from build123d import *

# Parameters (mm, degrees)
BOSS_EXTRUDE1_DEPTH   = 18
F_6_0MM_DOWEL_HOLE2_D = 9
SKETCH24_R            = 8.5
CUT_EXTRUDE7_DEPTH    = 19
CUT_EXTRUDE8_DEPTH    = 23
F_6_0MM_DOWEL_HOLE3_D = 9


with BuildPart() as part:
    # Sketch1 → Boss-Extrude1 (new body, symmetric)
    with BuildSketch(Plane.XY):
        with BuildLine():
            Line((-18.027756377, 6), (-22, 6))
            Line((-22, 6), (-22, 19))
            Line((-22, 19), (-50, 19))
            Line((-50, 19), (-50, 28))
            Line((-50, 28), (-25.690465157, 28))
            ThreePointArc((-25.690465157, 28), (-13.784048752, 35.411862419), (0, 38))
            Line((0, 38), (0, 19))
            ThreePointArc((0, 19), (-11.113055385, 15.411035007), (-18.027756377, 6))
        make_face()
    boss_extrude1 = extrude(amount=BOSS_EXTRUDE1_DEPTH, both=True)

    # Mirror1: Boss-Extrude1 across plane
    add(boss_extrude1.mirror(Plane(origin=(0, 0, 0), x_dir=(0, 0, 1), z_dir=(1, 0, 0))))

    # Ø6.0mm Dowel Hole2 (through all)
    with Locations(Plane(origin=(0, 28, 0), x_dir=(1, 0, 0), z_dir=(0, 1, 0))):
        with Locations((-31, 0)):
            Hole(F_6_0MM_DOWEL_HOLE2_D / 2)

    # Sketch24 → Cut-Extrude7 (cut)
    with BuildSketch(Plane(origin=(0, 28, 0), x_dir=(1, 0, 0), z_dir=(0, 1, 0))):
        with Locations((-31, 0)):
            Circle(SKETCH24_R)
    cut_extrude7 = extrude(amount=CUT_EXTRUDE7_DEPTH, mode=Mode.SUBTRACT)

    # Mirror5: Cut-Extrude7 across plane
    add(cut_extrude7.mirror(Plane(origin=(0, 0, 0), x_dir=(0, 0, 1), z_dir=(1, 0, 0))), mode=Mode.SUBTRACT)

    # Sketch25 → Cut-Extrude8 (cut, through all)
    with BuildSketch(Plane(origin=(0, 28, 0), x_dir=(1, 0, 0), z_dir=(0, 1, 0))):
        with BuildLine():
            Line((-44.497190923, 18), (-50, 18))
            Line((-50, 18), (-50, -18))
            Line((-50, -18), (-44.497190923, -18))
            ThreePointArc((-44.497190923, -18), (-48, 0), (-44.497190923, 18))
        make_face()
    cut_extrude8 = extrude(amount=-CUT_EXTRUDE8_DEPTH, mode=Mode.SUBTRACT)

    # Mirror7: Cut-Extrude8 across plane
    add(cut_extrude8.mirror(Plane(origin=(0, 0, 0), x_dir=(0, 0, 1), z_dir=(1, 0, 0))), mode=Mode.SUBTRACT)

    # Sketch28 → CBORE for M6 Hex Head Machine Screw1 (revolve, cut)
    with BuildSketch(Plane(origin=(-0.146360812, 37.999718137, 0), x_dir=(-0.999992583, -0.0038516, 0), z_dir=(0, 0, 1))):
        Polygon((0, 0), (0, 32.18492132), (2.5, 32.18492132), (2.5, 13.825), (3.325, 13), (3, 13), (3, 0), align=None)
    revolve(axis=Axis((-0.170818474, 44.349671037, 0), (0.0038516, -0.999992583, 0)), mode=Mode.SUBTRACT)

    # Ø6.0mm Dowel Hole3 (through all)
    with Locations(Plane(origin=(0, 28, 0), x_dir=(1, 0, 0), z_dir=(0, 1, 0))):
        with Locations((31, 0)):
            Hole(F_6_0MM_DOWEL_HOLE3_D / 2)


solid = part.part
Build history of the part. All positions in model axes, mm. A direction names the side the tool comes from. Give positions to 0.01 mm unless a question says otherwise; leave off trailing zeros. Order: outer loops, then holes, each group sorted by start corner. A loop starts at its lowest first (then second) coordinate and runs counter-clockwise, first axis right, second up. Notation, with made-up numbers: M 24.5,16.5 L 78.5,16.5 A15 ccw 78.5,45.5 Z; hole C 29,60.5 d8. An arc over 180 degrees is marked long. Put each result on its own line as item: value.
Item 1: Slice it at A-A, the plane x = -31. Write the cut outline in (y, z).
From the geometry:
outline: M 19,-18 L 28,-18 L 28,-4.5 L 19,-4.5 Z; M 19,4.5 L 28,4.5 L 28,18 L 19,18 Z
Item 2: Slice it at B-B, the plane z = 0. Give the number of separate pieces and of enclosed holes in the cut face, plus the area to 3 significant figures.
From the geometry:
separate pieces: 4
enclosed holes: 0
area: 1,170 mm2
Item 3: Flat gauge pins, fed straight in: pin 1 Ø8 at (x, z) = (8, 5.5) entering from +Y; pin 2 Ø1 at (y, z) = (22, 1.5) entering from +X; pin 3 Ø20.5 at (x, z) = (-30, -7) entering from +Y; pin 4 Ø8 at (x, y) = (-17.5, 34) entering from -Z. Where does each tip first touch, or does it go through?
From the geometry:
pin 1: stops at y = 37.79
pin 2: stops at x = 47.99
pin 3: stops at y = 32.46
pin 4: stops at z = -18
Item 4: Slice it at D-D, the plane z = 11. Write the cut outline in (x, y), plus the area to 3 significant figures.
From the geometry:
outline: M -46.72,19 L -22,19 L -22,6 L -18.03,6 A19 cw 18.03,6 L 22,6 L 22,19 L 46.72,19 L 46.72,28 L 25.69,28 A38 ccw -25.69,28 L -46.72,28 Z
area: 1,420 mm2
Item 5: 3-axis set-ups, long thin cutter, end or side, ignore diameter. For faces 1 (the cylindrical face through (22.5, 29, 0.1)), 2 (the flat face through (-22, 12, 0)), 3 (the flat face through (22, 12, 0)): which of +Z, -Z, +X, -X, +Y, -Y reach the whole face in a straight line?
From the geometry:
face 1: +X, +Y
face 2: +Z, -Z, -X, -Y
face 3: +Z, -Z, +X, -Y
Item 6: Slice it at C-C, the plane y = 11. Write the cut outline in (x, z), plus the area to 3 significant figures.
From the geometry:
outline: M -22,-18 L -15.49,-18 L -15.49,18 L -22,18 Z; M 15.49,-18 L 22,-18 L 22,18 L 15.49,18 Z
area: 469 mm2
Item 7: Probe line 1 (Z direction, x = 31, y = 21); line 2 (Y direction, x = -26.5, z = -7); line 3 (Y direction, x = -1, z = -3). List the from-to ranges inside material, lowest first. Write a range as [from, to].
From the geometry:
line 1: z = [-18, -4.5], [4.5, 18]
line 2: y = [19, 28]
line 3: y = [18.97, 24.8], [25, 37.99]
